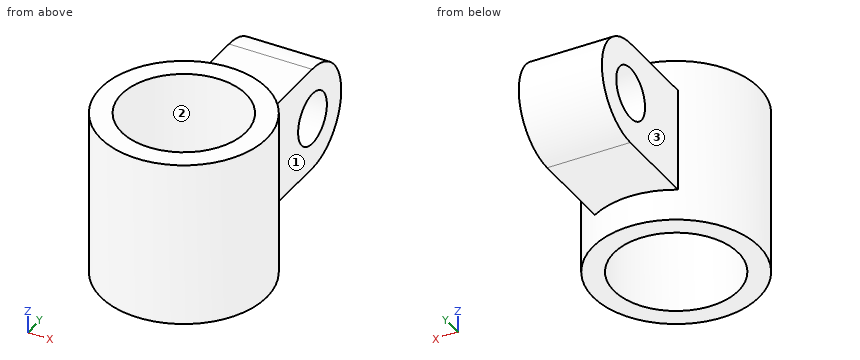
from build123d import *

# Parameters (mm, degrees)
F0_R          = 40
F1_DEPTH      = 80
F2_R          = 12.5
F3_DEPTH      = 20
F3_DEPTH_BACK = 20
F4_R          = 30
F5_DEPTH      = 146


with BuildPart() as f1:
    # F0 (on Top) → F1 (new body)
    with BuildSketch(Plane.XY):
        Circle(F0_R)
    extrude(amount=F1_DEPTH)

    # F2 (on Right) → F3 (join, two sides)
    with BuildSketch(Plane.YZ) as f3_sk:
        with BuildLine():
            Line((14.4573056011, 65.2065587372), (14.4573056011, 15.1210717529))
            Line((14.4573056011, 15.1210717529), (76.0508775141, 15.0012425378))
            ThreePointArc((76.0508775141, 15.0012425378), (100.7319009994, 40.3243347071), (75.40880883, 65.0053581924))
            Line((75.40880883, 65.0053581924), (14.4573056011, 65.2065587372))
        make_face()
        with Locations((75.7298431721, 40.0033003651)):
            Circle(F2_R, mode=Mode.SUBTRACT)
    extrude(amount=-F3_DEPTH)
    extrude(f3_sk.sketch, amount=F3_DEPTH_BACK)

    # F4 (on face) → F5 (cut)
    with BuildSketch(Plane.XY.offset(80)):
        Circle(F4_R)
    extrude(amount=-F5_DEPTH, mode=Mode.SUBTRACT)


solid = f1.part
The model under review builds one solid part; all positions refer to its coordinate system, in mm. Face numbers are marked on the shaded views. Round coordinates to 2 decimals unless told otherwise and drop trailing zeros. Loops run counter-clockwise (first coordinate to the right, second up) from the corner with the lowest first, then second, coordinate; pieces in that order, holes last. Notation, with made-up numbers: M -15,40 L 8,40 A18 ccw 8,56 Z; hole C 56.5,3.25 d2. An arc over 180 degrees is marked long. Answer as CSV lines item,"result". Start each with the question number.
Item 1: Consider section D-D (x = 25). Write out the cut boundary in (y, z).
Item 2: Wall thickness on line 1 (Y direction, x = 0, z = 47); line 2 (X direction, y = 15, z = 31); line 3 (X direction, y = 7, z = 43): over which ranges is each line inside the solid? List them lowest first. Write a range as [from, to].
Item 3: Mouldability with a two-part tool opening along X and no side actions: class the marked faces 1, 2 and 3 as released by +X, released by -X, zero draft, split by the parting line, or undercut.
Item 4: Consider section C-C (y = 0). Write out the cut boundary in (x, z).
Item 5: Consider section B-B (z = 35.5). Write out the cut boundary in (x, y), then the cut area to 3 significant figures.
Item 6: Insertion check: P1, Ø3, axis at x = -21, y = 60.5, coming from the -Z side; P2, Ø6, axis at x = -6, z = 22, coming from the +Y side; P3, Ø6, axis at x = -16, z = 10.5, coming from the +Y side. Each pin has a flat end and moves straight along its axis. Give the tip position at first contact, or say it passes through.
Item 7: Consider section A-A (x = -7). Write out the cut boundary in (y, z), then the cut area to 3 significant figures.
Answer:
1,outline,"M -31.22,0 L -16.58,0 L -16.58,80 L -31.22,80 Z; M 16.58,0 L 31.22,0 L 31.22,80 L 16.58,80 Z"
2,line 1,"y = [-40, -30], [30, 65.37], [86.09, 99.74]"
2,line 2,"x = [-37.08, -25.98], [25.98, 37.08]"
2,line 3,"x = [-39.38, -29.17], [29.17, 39.38]"
3,face 1,"released by +X"
3,face 2,"undercut"
3,face 3,"released by -X"
4,outline,"M -40,0 L -30,0 L -30,80 L -40,80 Z; M 30,0 L 40,0 L 40,80 L 30,80 Z"
5,outline,"M -20,34.64 A40 ccw long 20,34.64 L 20,64.07 L -20,64.07 Z; M -20,87.39 L 20,87.39 L 20,100.33 L -20,100.33 Z; hole C 0,0 d60"
5,area,"3,750 mm^2"
6,P1,"stops at z = 15.03"
6,P2,"stops at y = 95.73"
6,P3,"stops at y = 37.83"
7,outline,"M -39.38,0 L -29.17,0 L -29.17,80 L -39.38,80 Z; M 29.17,0 L 39.38,0 L 39.38,15.07 L 76.05,15 A25 ccw 75.41,65.01 L 39.38,65.12 L 39.38,80 L 29.17,80 Z; hole C 75.73,40 d25"
7,area,"3,940 mm^2"
